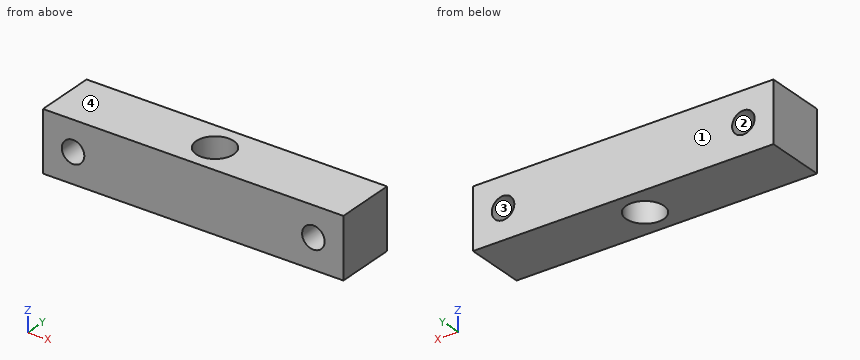
```python
from build123d import *

# Parameters (mm, degrees)
BOX_W           = 40
BOX_H           = 8
BOX_DEPTH       = 8
SKETCH_R        = 2.5
POCKET_DEPTH    = 8
SKETCH001_R     = 1.5
POCKET001_DEPTH = 8


with BuildPart() as part:
    # Box → Box (new body)
    with BuildSketch(Plane(origin=(-20, -4, -4), x_dir=(1, 0, 0), z_dir=(0, 0, 1))):
        with Locations((20, 4)):
            Rectangle(BOX_W, BOX_H)
    extrude(amount=BOX_DEPTH)

    # Sketch → Pocket (cut)
    with BuildSketch(Plane(origin=(-20, -4, 4), x_dir=(1, 0, 0), z_dir=(0, 0, 1))):
        with Locations((20, 4)):
            Circle(SKETCH_R)
    extrude(amount=-POCKET_DEPTH, mode=Mode.SUBTRACT)

    # Sketch001 → Pocket001 (cut)
    with BuildSketch(Plane(origin=(-20, -4, -4), x_dir=(1, 0, 0), z_dir=(0, -1, 0))):
        with Locations((4, 4)):
            Circle(SKETCH001_R)
        with Locations((36, 4)):
            Circle(SKETCH001_R)
    extrude(amount=-POCKET001_DEPTH, mode=Mode.SUBTRACT)


solid = part.part
```
The model under review builds one solid part; all positions refer to its coordinate system, in mm. Face numbers are marked on the shaded views. Give positions to 0.01 mm unless a question says otherwise; leave off trailing zeros. Write each loop counter-clockwise with the first axis right and the second up, starting at its lowest first coordinate (ties: lowest second). Pieces come first, ordered by that corner, then holes. Notation, with made-up numbers: (31, 15.25) -> (55, 15.25) arc R12 cw to (55, 31.25) -> close; hole circle Ø1 at (89, -26). An arc over 180 degrees is marked (long way). Put each result on its own line as item: value.
(1) We need section C-C, the plane y = 1.75. Give the boundary of the cut face in (x, z).
Results are:
outline: (-20, -4) -> (-1.79, -4) -> (-1.79, 4) -> (-20, 4) -> close; (1.79, -4) -> (20, -4) -> (20, 4) -> (1.79, 4) -> close; hole circle Ø3 at (-16, 0); hole circle Ø3 at (16, 0)
(2) We need section A-A, the plane z = 0. Give the boundary of the cut face in (x, y), and give its area (3 significant figures).
Results are:
outline: (-20, -4) -> (-17.5, -4) -> (-17.5, 4) -> (-20, 4) -> close; (-14.5, -4) -> (14.5, -4) -> (14.5, 4) -> (-14.5, 4) -> close; (17.5, -4) -> (20, -4) -> (20, 4) -> (17.5, 4) -> close; hole circle Ø5 at (0, 0)
area: 252 mm²
(3) We need section B-B, the plane x = 16. Give the boundary of the cut face in (y, z), and give its area (3 significant figures).
Results are:
outline: (-4, -4) -> (4, -4) -> (4, -1.5) -> (-4, -1.5) -> close; (-4, 1.5) -> (4, 1.5) -> (4, 4) -> (-4, 4) -> close
area: 40.0 mm²
(4) The part is to be moulded in two halves that separate along Z. For the marked faces 1, 2, 3 and 4, say which applies: pulls with the +Z half, pulls with the -Z half, needs draft (parallel to the pull), parting line crosses it, or undercut.
Results are:
face 1: needs draft
face 2: undercut
face 3: undercut
face 4: pulls with the +Z half
(5) For pin 1 Ø1 at (x, z) = (15.5, 0) entering from -Y, flat-tipped, find the tip position at first contact; note if it passes through.
Results are:
pin 1: through
(6) To check wall thickness, follow probe 1 along Y at (x, z) = (0, 0.75); probe 2 along Z at (x, y) = (16, 0.75); probe 3 along X at (y, z) = (-1.25, 0.5). State the ranges of each line that lie inside material, in increasing order. Write a range as from..to.
Results are:
probe 1: -4..-2.5, 2.5..4
probe 2: -4..-1.5, 1.5..4
probe 3: -20..-17.41, -14.59..-2.17, 2.17..14.59, 17.41..20
(7) We need section D-D, the plane y = 3.25. Give the boundary of the cut face in (x, z).
Results are:
outline: (-20, -4) -> (20, -4) -> (20, 4) -> (-20, 4) -> close; hole circle Ø3 at (-16, 0); hole circle Ø3 at (16, 0)
